Source: CAD feature listing. Evaluate the final solid. Frame: model axes, mm. A direction names the side the tool comes from. Coordinates: 2 decimals unless noted, no trailing zeros. Write each loop counter-clockwise with the first axis right and the second up, starting at its lowest first coordinate (ties: lowest second). Pieces come first, ordered by that corner, then holes. Notation, with made-up numbers: M -21.5,10 L 21.5,10 A34 ccw 21.5,48 Z; hole C -28.5,53.25 d10. An arc over 180 degrees is marked long. Write item = value, one per line. Start each with the question number.
1. Section query A-A (z = -13.25). Output: boundary loops of the cut face in (x, y).
2. Section query C-C (y = 3). Output: boundary loops of the cut face in (x, z).
3. Pull-direction query (X, two-part tool) for faces 1 (the face through (2.726, 25.567, -14.164)), 2 (the face through (-1, 25.8, -14)), 3 (the face through (4.5, 18, -3)); classes: pulls with the +X half, pulls with the -X half, needs draft (parallel to the pull), parting line crosses it, or undercut.
4. Pin query (flat end, axial travel): pin 1 Ø1.5 at (x, y) = (-0.5, 25) entering from +Z; pin 2 Ø3 at (y, z) = (27, -13.25) entering from +X; pin 3 Ø5 at (x, z) = (-2.5, 3.5) entering from +Y. Return the tip coordinate at first contact, or that it passes through.
5. Section query B-B (x = 1.5). Output: boundary loops of the cut face in (y, z), then the cut area to 3 significant figures.
6. Section query D-D (z = 4.5). Output: boundary loops of the cut face in (x, y), then the cut area to 3 significant figures.
7. Line query: line 1 along Z through (x, y) = (-2.9, 3); line 2 along Y through (x, z) = (-0.9, 4.5); line 3 along X through (y, z) = (27, -8.25). Output: solid intervals per line, ascending.
8. Access query for faces 4 (the face through (0, 30, -4)), 5 (the face through (-2, 6, 3)), 6 (the face through (-1, 23, -5)). Directions: +Z, -Z, +X, -X, +Y, -Y. A direction counts if a zero-diameter tool reaches every point of the face in a straight line with its end or side. Return the directions, or none.
Autodesk Inventor part; units mm, degrees
ref_plane "Work Plane1" through (0, 0, 0) normal (-1, 0, 0) x (0, 0, 1)
ref_plane "YZ Plane" through (0, 0, 0) normal (1, 0, 0) x (0, 1, 0)
ref_plane "XZ Plane" through (0, 0, 0) normal (0, 1, 0) x (-1, 0, 0)
sketch "Sketch1" plane through (0, 0, 0) normal (1, 0, 0) x (0, 1, 0)
  line L0 (0, 0) -> (30, 0)
  line L1 (30, 0) -> (30, -3.5)
  line L2 (30, -3.5) -> (0, -3.5)
  line L3 (0, -3.5) -> (0, 0)
  dimension "d0" = 3.5
  dimension "d1" = 30
extrude "Extrusion1" add sketch "Sketch1" along normal mid plane 9
sketch "Sketch2" plane through (-4.5, 0, -3.5) normal (0, 0, -1) x (-1, 0, 0)
  line L0 (-9, 30) -> (0, 30)
  line L1 (0, 0) -> (0, 30)
  line L2 (-9, 30) -> (0, 30)
  line L3 (0, 30) -> (0, 23)
  line L4 (0, 23) -> (-9, 23)
  line L5 (-9, 23) -> (-9, 30)
  point P0 (-4.5, 0)
  dimension "d4" = 7
extrude "Extrusion2" add sketch "Sketch2" along normal blind 12.25
ref_plane "Work Plane1" through (0, 0, 0) normal (-1, 0, 0) x (0, 0, 1)
sketch "Sketch3" plane through (-4.5, 0, 0) normal (0, 0, 1) x (1, 0, 0)
  line L0 (4.5, 0) -> (9, 0)
  line L1 (0, 0) -> (4.5, 0)
  line L2 (4.5, 0) -> (4.5, 6)
  line L3 (4.5, 6) -> (0, 6)
  line L4 (0, 6) -> (0, 0)
  line L5 (9, 30) -> (0, 30)
  line L6 (4.5, -6) -> (4.5, 36)
  point P0 (4.5, 30)
  dimension "d7" = 4.5
  dimension "d8" = 4.5
  dimension "d9" = 6
extrude "Extrusion3" add sketch "Sketch3" along normal blind 6
sketch "Sketch7" plane through (-4.5, 30, 0) normal (0, 1, 0) x (1, 0, 0)
  circle A0 centre (4.5, 8.25) radius 3.2004
  line L0 (0, 15.75) -> (9, 15.75)
  point P0 (4.5, 0)
  dimension "d42" = 6.4008
  dimension "d43" = 7.5
extrude "Extrusion6" cut sketch "Sketch7" against normal up to next
sketch "Sketch8" plane through (-4.5, 30, 0) normal (0, 1, 0) x (1, 0, 0)
  line L0 (9, 15.75) -> (0, 15.75)
  line L1 (5.5, 7.75) -> (3.5, 7.75)
  line L2 (3.5, 7.75) -> (3.5, 15.75)
  line L3 (3.5, 15.75) -> (5.5, 15.75)
  line L4 (5.5, 15.75) -> (5.5, 7.75)
  line L5 (5.5, 7.75) -> (3.5, 15.75) construction
  line L6 (3.5, 7.75) -> (5.5, 15.75) construction
  line L7 (4.5, -3.15) -> (4.5, 18.9)
  point P0 (4.5, 0)
  point P1 (4.5, 11.75)
  dimension "d46" = 8
  dimension "d47" = 2
  dimension "d48" = 1
extrude "Extrusion7" cut sketch "Sketch8" against normal up to next
sketch "Sketch9" plane through (4.5, 0, 0) normal (1, 0, 0) x (0, 0, -1)
  line L0 (0, 30) -> (15.75, 30)
  line L1 (15.75, 30) -> (15.75, 23)
  point P0 (0, 0)
  point P1 (13.25, 27)
  dimension "d51" = 3
  dimension "d52" = 2.5
hole "Hole2" at (4.5, 27, -13.25) direction (-1, 0, 0) diameter 3.4 depth 3.5
sketch "Sketch10" plane through (-1, 30, -11.2902) normal (1, 0, 0) x (0, 0, -1)
  circle A0 centre (1.9598, -3) radius 1.7
  point P0 (-11.2902, -30)
  point P1 (3.0161, 3.0772)
hole "Hole3" at (-1, 27, -13.25) direction (-1, 0, 0) diameter 2.459 depth 3.5
chamfer "Chamfer1" distance 3 angle 45 2 edges at (2.75, 23, -15.75) (-2.75, 23, -15.75)
sketch "Sketch13" plane through (0, 0, 0) normal (1, 0, 0) x (0, 0, -1)
  line L0 (0, 0) -> (-6, 0)
  line L1 (-6, 0) -> (-6, 6)
  line L2 (0, 6) -> (-6, 6)
  line L3 (0, 30) -> (0, 0)
  point P0 (-4.5, 3)
  dimension "d91" = 3
  dimension "d92" = 4.5
hole "Hole4" at (0, 3, 4.5) direction (-1, 0, 0) diameter 1.567 end through all
sketch "Sketch14" plane through (0, 0, 0) normal (1, 0, 0) x (0, 0, -1)
  line L0 (-6, 0) -> (-6, 6)
  line L1 (0, 6) -> (-6, 6)
  point P0 (0, 0)
  point P1 (-1.5, 3)
  dimension "d100" = 4.5
  dimension "d101" = 3
hole "Hole5" at (0, 3, 1.5) direction (-1, 0, 0) diameter 1.567 end through all
properties part number "MEM to dovetail rod adapter - v3"
Results are:
q1.outline = M -4.5,23.5 L -1,23.5 L -1,25.77 L -4.5,25.77 Z; M -4.5,28.23 L -1,28.23 L -1,30 L -4.5,30 Z; M 1,23.5 L 4.5,23.5 L 4.5,25.3 L 1,25.3 Z; M 1,28.7 L 4.5,28.7 L 4.5,30 L 1,30 Z
q2.outline = M -4.5,-3.5 L 4.5,-3.5 L 4.5,0 L 0,0 L 0,0.72 L -4.5,0.72 Z; M -4.5,2.28 L 0,2.28 L 0,3.72 L -4.5,3.72 Z; M -4.5,5.28 L 0,5.28 L 0,6 L -4.5,6 Z
q3.face_1 = needs draft
q3.face_2 = undercut
q3.face_3 = pulls with the +X half
q4.pin_1 = 0
q4.pin_2 = -1
q4.pin_3 = 6
q5.outline = M 0,-3.5 L 23,-3.5 L 23,-5.42 L 30,-5.42 L 30,0 L 0,0 Z; M 23,-12.75 L 26,-15.75 L 30,-15.75 L 30,-11.08 L 23,-11.08 Z; hole C 27,-13.25 d3.4
q5.area = 138 mm^2
q6.outline = M -4.5,0 L 0,0 L 0,2.22 L -4.5,2.22 Z; M -4.5,3.78 L 0,3.78 L 0,6 L -4.5,6 Z
q6.area = 19.9 mm^2
q7.line_1 = -3.5 to 0.72, 2.28 to 3.72, 5.28 to 6
q7.line_2 = 0 to 2.22, 3.78 to 6
q7.line_3 = -4.5 to -3.2, 3.2 to 4.5
q8.face_4 = +Z, -Z, +X, -X, +Y
q8.face_5 = +Z, +X, -X, +Y
q8.face_6 = -Z, +X, -X, -Y
